from build123d import *

# Parameters (mm, degrees)
CBORE_FOR_1_4_BINDING_HEAD_MACHINE_SCREW_D           = 6.5278
CBORE_FOR_1_4_BINDING_HEAD_MACHINE_SCREW_DEPTH       = 303
CBORE_FOR_1_4_BINDING_HEAD_MACHINE_SCREW_CBORE_D     = 14.2875
CBORE_FOR_1_4_BINDING_HEAD_MACHINE_SCREW_CBORE_DEPTH = 9.525
CBORE_FOR_1_4_BINDING_HEAD_MACHINE_SCREW_TIP         = 1.961148974


with BuildPart() as part:
    # Sketch1 → Revolve1 (revolve)
    with BuildSketch(Plane.XY, mode=Mode.PRIVATE) as revolve1_sk:
        Polygon((0, 0), (0, 8.5), (11, 8.5), (11, 14), (15, 14), (15, 0), align=None)
    revolve(revolve1_sk.sketch.rotate(Axis((0, 0, 0), (-1, 0, 0)), 90), axis=Axis((0, 0, 0), (-1, 0, 0)))

    # CBORE for 1/4 Binding Head Machine Screw1
    with Locations(Plane(origin=(15, 0, 0), x_dir=(0, 0, -1), z_dir=(1, 0, 0))):
        with Locations((0, 0)):
            CounterBoreHole(CBORE_FOR_1_4_BINDING_HEAD_MACHINE_SCREW_D / 2, CBORE_FOR_1_4_BINDING_HEAD_MACHINE_SCREW_CBORE_D / 2, CBORE_FOR_1_4_BINDING_HEAD_MACHINE_SCREW_CBORE_DEPTH, depth=CBORE_FOR_1_4_BINDING_HEAD_MACHINE_SCREW_DEPTH)
            with Locations((0, 0, -(CBORE_FOR_1_4_BINDING_HEAD_MACHINE_SCREW_DEPTH + CBORE_FOR_1_4_BINDING_HEAD_MACHINE_SCREW_TIP / 2))):  # 118° drill point
                Cone(0, CBORE_FOR_1_4_BINDING_HEAD_MACHINE_SCREW_D / 2, CBORE_FOR_1_4_BINDING_HEAD_MACHINE_SCREW_TIP, mode=Mode.SUBTRACT)


solid = part.part
Could you check a few things on this model? Use its own coordinates, in mm. A direction names the side the tool comes from. Coordinates: 2 decimals unless noted, no trailing zeros. Loops run counter-clockwise (first coordinate to the right, second up) from the corner with the lowest first, then second, coordinate; pieces in that order, holes last. Notation, with made-up numbers: (58, 39.5) -> (68, 39.5) arc R22 ccw to (68, 49.5) -> close; hole circle Ø2 at (-3, 32.5). An arc over 180 degrees is marked (long way). Answer in a Markdown table with one row per item.
(1) Imagine slicing it at C-C (x = 3.25). List the corners of the cut face in (y, z) for me.
Results found:
| item | result |
|---|---|
| outline | circle Ø17 at (0, 0); hole circle Ø6.53 at (0, 0) |
(2) For faces 1 (the face through (5.577, -8.428, 1.107)), 2 (the face through (10.304, 0.314, 7.137)), 3 (the face through (0, 0, 4)), which set-ups out of +Z, -Z, +X, -X, +Y, -Y let a thin tool reach every point of the face, with its end or its side?
Results found:
| item | result |
|---|---|
| face 1 | -X |
| face 2 | +X |
| face 3 | +Z, -Z, -X, +Y, -Y |
(3) Will these pins go through, and if not, where does the flat tip stop? pin 1 Ø6 at (x, z) = (10.5, -3.5) entering from +Y; pin 2 Ø4.5 at (y, z) = (3, 1) entering from +X (3 decimals); pin 3 Ø5 at (y, z) = (-4.5, 5) entering from -X; pin 4 Ø5 at (x, y) = (11.5, 4.5) entering from +Z.
Results found:
| item | result |
|---|---|
| pin 1 | stops at y = 13.99 |
| pin 2 | stops at x = 5.475 |
| pin 3 | stops at x = 0 |
| pin 4 | stops at z = 13.86 |
(4) Imagine slicing it at D-D (y = 4.5). List the corners of the cut face in (x, z) for me (3 decimals), plus the area to 3 significant figures.
Results found:
| item | result |
|---|---|
| outline | (0, -7.211) -> (11, -7.211) -> (11, -13.257) -> (15, -13.257) -> (15, -5.548) -> (5.475, -5.548) -> (5.475, 5.548) -> (15, 5.548) -> (15, 13.257) -> (11, 13.257) -> (11, 7.211) -> (0, 7.211) -> close |
| area | 159 mm^2 |
(5) Imagine slicing it at A-A (z = 0). List the corners of the cut face in (x, y) for me (3 decimals), plus the area to 3 significant figures.
Results found:
| item | result |
|---|---|
| outline | (0, -8.5) -> (11, -8.5) -> (11, -14) -> (15, -14) -> (15, -7.144) -> (5.475, -7.144) -> (5.475, -3.264) -> (0, -3.264) -> close; (0, 3.264) -> (5.475, 3.264) -> (5.475, 7.144) -> (15, 7.144) -> (15, 14) -> (11, 14) -> (11, 8.5) -> (0, 8.5) -> close |
| area | 127 mm^2 |
(6) Thinking about a two-plate mould opening in Y: for faces 4 (the face through (11, 9, 0)), 5 (the face through (13, 12.4, -6.5)), 6 (the face through (5.475, -1.5, -3.1)), which applies, released by +Y, released by -Y, zero draft, split by the parting line, or undercut?
Results found:
| item | result |
|---|---|
| face 4 | zero draft |
| face 5 | split by the parting line |
| face 6 | undercut |
(7) If I drill on probe 1 along Y at (x, z) = (4.3, 0); probe 2 along Y at (x, z) = (10, 0); probe 3 along X at (y, z) = (-11.5, 6.75), over which ranges is the centre line in solid material (lowest first)?
Results found:
| item | result |
|---|---|
| probe 1 | y = -8.5 to -3.26, 3.26 to 8.5 |
| probe 2 | y = -8.5 to -7.14, 7.14 to 8.5 |
| probe 3 | x = 11 to 15 |
